from build123d import *

# Parameters (mm, degrees)
F0_R     = 12.7
F1_DEPTH = 76.2
F2_R     = 12.7
F4_DEPTH = 50.8


with BuildPart() as f1:
    # F0 (on Top) → F1 (new body)
    with BuildSketch(Plane.XY):
        Circle(F0_R)
    extrude(amount=F1_DEPTH)

    # F2
    f2_edges = [f1.edges().sort_by_distance(p)[0] for p in [
        (-12.7, 0, 76.2),
    ]]
    fillet(f2_edges, radius=F2_R)

    # F3 (on Front) → F4 (cut)
    with BuildSketch(Plane.XZ):
        Polygon((-6.35, 37.873212), (0, 37.873212), (6.35, 37.873212), (6.35, 50.573212), (-6.35, 50.573212), align=None)
    extrude(amount=F4_DEPTH, mode=Mode.SUBTRACT)


solid = f1.part
Model file for the job. Use its own axes, mm. Give positions to 0.01 mm unless a question says otherwise; leave off trailing zeros. Loops run counter-clockwise (first coordinate to the right, second up) from the corner with the lowest first, then second, coordinate; pieces in that order, holes last.
Item 1: Slice it at A-A (x = 0). Write the cut outline in (y, z), plus the area to 3 significant figures.
Check values:
outline: (-12.7, 0) - (12.7, 0) - (12.7, 63.5) arc R12.7 ccw to (-12.7, 63.5) - (-12.7, 50.57) - (0, 50.57) - (0, 37.87) - (-12.7, 37.87) - close
area: 1,700 mm2
Item 2: Slice it at D-D (x = 3.75). Write the cut outline in (y, z), plus the area to 3 significant figures.
Check values:
outline: (-12.13, 0) - (12.13, 0) - (12.13, 63.5) arc R12.13 ccw to (-12.13, 63.5) - (-12.13, 50.57) - (0, 50.57) - (0, 37.87) - (-12.13, 37.87) - close
area: 1,620 mm2
Item 3: Slice it at B-B (y = -8). Write the cut outline in (x, z), plus the area to 3 significant figures.
Check values:
outline: (-9.86, 0) - (9.86, 0) - (9.86, 63.5) arc R9.86 ccw to (-9.86, 63.5) - close; hole (-6.35, 37.87) - (6.35, 37.87) - (6.35, 50.57) - (-6.35, 50.57) - close
area: 1,240 mm2
Item 4: Drop flat-ended pins along their axis: P1, Ø3.5, axis at y = -3, z = 45.5, coming from the -X side; P2, Ø10, axis at x = -1, y = -6, coming from the +Z side; P3, Ø1.5, axis at y = 5.5, z = 57.5, coming from the +X side. Give the stop position or say it passes through.
Check values:
P1: stops at x = -12.64
P2: stops at z = 76.15
P3: stops at x = 11.78
Item 5: Mould opens along X. For faces 1 (the face through (-1.653, 12.592, 31.306)), 2 (the face through (0, 0, 0)), 3 (the face through (-6.35, -5, 44)) say: +X half, -X half, draft (parallel to the pull), parting line (faces both ways), or undercut.
Check values:
face 1: parting line
face 2: draft
face 3: undercut
Item 6: Drill centre lines: line 1 along Y through (x, z) = (0, 44.5); line 2 along Z through (x, y) = (-3.5, -8.5); line 3 along X through (y, z) = (-7.25, 44). Where is each one in solid material? Low to high.
Check values:
line 1: y = 0 to 12.7
line 2: z = 0 to 37.87, 50.57 to 72.26
line 3: x = -10.43 to -6.35, 6.35 to 10.43
Item 7: Slice it at C-C (z = 60.5). Write the cut outline in (x, y), plus the area to 3 significant figures.
Check values:
outline: circle Ø25.4 at (0, 0)
area: 507 mm2
